```python
from build123d import *

# Parameters (mm, degrees)
SKETCH2_R           = 50
BOSS_EXTRUDE1_DEPTH = 10
SKETCH1_R           = 1
SKETCH1_R_2         = 2
CUT_EXTRUDE2_DEPTH  = 72.414284285
CUT_EXTRUDE3_START  = -10
SKETCH3_R           = 3
CUT_EXTRUDE3_DEPTH  = 62.414284285


with BuildPart() as part:
    # Sketch2 → Boss-Extrude1 (new body)
    with BuildSketch(Plane.XY):
        Circle(SKETCH2_R)
        with BuildLine():
            Line((2.5, 39.921798557), (2.5, 3.122498999))
            ThreePointArc((2.5, 3.122498999), (3.464101615, 2), (3.954163457, 0.60381401))
            Line((3.954163457, 0.60381401), (35.823291715, -17.795835769))
            ThreePointArc((35.823291715, -17.795835769), (34.641016151, 20), (2.5, 39.921798557))
        make_face(mode=Mode.SUBTRACT)
        with BuildLine():
            Line((-2.5, 39.921798557), (-2.5, 3.122498999))
            ThreePointArc((-2.5, 3.122498999), (-3.464101615, 2), (-3.954163457, 0.60381401))
            Line((-3.954163457, 0.60381401), (-35.823291715, -17.795835769))
            ThreePointArc((-35.823291715, -17.795835769), (-34.641016151, 20), (-2.5, 39.921798557))
        make_face(mode=Mode.SUBTRACT)
        with BuildLine():
            Line((33.323291715, -22.125962788), (1.454163457, -3.726313009))
            ThreePointArc((1.454163457, -3.726313009), (0, -4), (-1.454163457, -3.726313009))
            Line((-1.454163457, -3.726313009), (-33.323291715, -22.125962788))
            ThreePointArc((-33.323291715, -22.125962788), (0, -40), (33.323291715, -22.125962788))
        make_face(mode=Mode.SUBTRACT)
    extrude(amount=BOSS_EXTRUDE1_DEPTH)

    # Sketch1 → Cut-Extrude2 (cut, through all)
    with BuildSketch(Plane.XY):
        with Locations((0, 10)):
            Circle(SKETCH1_R)
        Circle(SKETCH1_R_2)
        with Locations((-8.660254038, -5)):
            Circle(SKETCH1_R)
        with Locations((8.660254038, -5)):
            Circle(SKETCH1_R)
    extrude(amount=CUT_EXTRUDE2_DEPTH, mode=Mode.SUBTRACT)

    # Sketch3 → Cut-Extrude3 (cut, through all)
    with BuildSketch(Plane(origin=(0, 0, 0), x_dir=(1, 0, 0), z_dir=(0, 1, 0)).offset(CUT_EXTRUDE3_START)):
        with Locations(Location((0, -5, 0), (0, 0, 270))):
            Circle(SKETCH3_R)
    extrude(amount=-CUT_EXTRUDE3_DEPTH, mode=Mode.SUBTRACT)


solid = part.part
```
For this review, take the finished solid that the model builds, in its own axes (mm). A direction names the side the tool comes from. Round coordinates to 2 decimals unless told otherwise and drop trailing zeros. Write each loop counter-clockwise with the first axis right and the second up, starting at its lowest first coordinate (ties: lowest second). Pieces come first, ordered by that corner, then holes. Notation, with made-up numbers: (35.25, -3.75) -> (45.25, -3.75) arc R8 cw to (45.25, 9.25) -> close; hole circle Ø3 at (-12, 57.5). An arc over 180 degrees is marked (long way). One line per question, with ' | ' between items. Start each with the question number.
(1) For line 1 along Y through (x, z) = (0, 6.75); line 2 along Y through (x, z) = (-27, 4.75); line 3 along X through (y, z) = (4, 1.75), list the stretches that pass through material, from the lowest coordinate up. Write a range as from..to.
(2) Add section A-A, the plane x = -15.5. Write out the cut boundary in (y, z).
(3) Add section D-D, the plane y = -8.5. Write out the cut boundary in (x, z).
(4) Add section B-B, the plane y = 5. Write out the cut boundary in (x, z), plus the area to 3 significant figures.
(5) Insertion check: P1, Ø1.5, axis at y = -39.5, z = 5, coming from the +X side; P2, Ø1, axis at x = -23.5, z = 6.5, coming from the +Y side; P3, Ø2, axis at x = -26.5, y = -36, coming from the -Z side; P4, Ø5, axis at x = 0, z = 5, coming from the +Y side. Each pin has a flat end and moves straight along its axis. Give the tip position at first contact, or say it passes through.
(6) Mouldability with a two-part tool opening along Y and no side actions: class faces 4 (the face through (-1, 12, 0)), 5 (the face through (19.67, -8.47, 4.93)), 6 (the face through (47.69, 15.02, 4.93)) as released by +Y, released by -Y, zero draft, split by the parting line, or undercut.
(7) Add section C-C, the plane z = 3.5. Write out the cut boundary in (x, y).
(8) Tool access review of faces 1 (the face through (0, -45, 2)), 2 (the face through (17.612, -13.055, 4.93)), 3 (the face through (-1, 12, 10)): name each direction out of +Z, -Z, +X, -X, +Y, -Y from which nothing blocks a thin tool from reaching the whole face with its end or side.
Answer list:
1) line 1: -4..-2, 2..9, 11..50 | line 2: -42.08..-29.51, -18.48..-12.7, 29.51..42.08 | line 3: -49.84..-39.8, -2.5..2.5, 39.8..49.84
2) outline: (-47.54, 0) -> (-36.87, 0) -> (-36.87, 10) -> (-47.54, 10) -> close; (-11.84, 0) -> (-6.06, 0) -> (-6.06, 10) -> (-11.84, 10) -> close; (36.87, 0) -> (47.54, 0) -> (47.54, 10) -> (36.87, 10) -> close
3) outline: (-49.27, 0) -> (-39.09, 0) -> (-39.09, 10) -> (-49.27, 10) -> close; (-19.72, 0) -> (-9.72, 0) -> (-9.72, 10) -> (-19.72, 10) -> close; (9.72, 0) -> (19.72, 0) -> (19.72, 10) -> (9.72, 10) -> close; (39.09, 0) -> (49.27, 0) -> (49.27, 10) -> (39.09, 10) -> close
4) outline: (-49.75, 0) -> (-39.69, 0) -> (-39.69, 10) -> (-49.75, 10) -> close; (-2.5, 0) -> (2.5, 0) -> (2.5, 10) -> (-2.5, 10) -> close; (39.69, 0) -> (49.75, 0) -> (49.75, 10) -> (39.69, 10) -> close | area: 251 mm²
5) P1: x = 31.6 | P2: y = 44.4 | P3: z = 0 | P4: y = 50
6) face 4: zero draft | face 5: undercut | face 6: split by the parting line
7) outline: (-33.32, -22.13) -> (-1.45, -3.73) arc R4 ccw to (1.45, -3.73) -> (33.32, -22.13) arc R40 cw to (2.6, -39.92) -> (2.6, -49.93) arc R50 ccw (long way) to (-2.6, -49.93) -> (-2.6, -39.92) arc R40 cw to start; hole (-35.82, -17.8) -> (-3.95, 0.6) arc R4 cw to (-2.5, 3.12) -> (-2.5, 39.92) arc R40 ccw to start; hole circle Ø2 at (-8.66, -5); hole circle Ø4 at (0, 0); hole circle Ø2 at (0, 10); hole (2.5, 3.12) arc R4 cw to (3.95, 0.6) -> (35.82, -17.8) arc R40 ccw to (2.5, 39.92) -> close; hole circle Ø2 at (8.66, -5)
8) face 1: -Y | face 2: +Z, -Z | face 3: +Z, +X, -X, +Y, -Y
